from build123d import *

# Parameters (mm, degrees)
CROQUIS1_R              = 12
CROQUIS1_R_2            = 1.7
SALIENTE_EXTRUIR1_DEPTH = 10
CROQUIS2_R              = 4
SALIENTE_EXTRUIR2_DEPTH = 20
CORTAR_EXTRUIR1_REACH   = 12
CROQUIS3_R              = 5.5


with BuildPart() as part:
    # Croquis1 → Saliente-Extruir1 (new body)
    with BuildSketch(Plane.XY):
        Circle(CROQUIS1_R)
        with Locations((-5.655, 5.655)):
            Circle(CROQUIS1_R_2, mode=Mode.SUBTRACT)
        with Locations((5.655, 5.655)):
            Circle(CROQUIS1_R_2, mode=Mode.SUBTRACT)
        with Locations((5.655, -5.655)):
            Circle(CROQUIS1_R_2, mode=Mode.SUBTRACT)
        with Locations((-5.655, -5.655)):
            Circle(CROQUIS1_R_2, mode=Mode.SUBTRACT)
    extrude(amount=SALIENTE_EXTRUIR1_DEPTH)

    # Croquis2 → Saliente-Extruir2 (add, symmetric)
    with BuildSketch(Plane(origin=(0, 0, 0), x_dir=(0, 0, -1), z_dir=(1, 0, 0))):
        with Locations((-4, 0)):
            Circle(CROQUIS2_R)
    extrude(amount=SALIENTE_EXTRUIR2_DEPTH, both=True)

    # Croquis3 → Cortar-Extruir1 (cut, up to next)
    with BuildSketch(Plane.XY.offset(10), mode=Mode.PRIVATE) as cortar_extruir1_sk1:
        Circle(CROQUIS3_R)
    cortar_extruir1_tool1 = extrude(cortar_extruir1_sk1.sketch, amount=-CORTAR_EXTRUIR1_REACH, mode=Mode.PRIVATE) & part.part
    add(cortar_extruir1_tool1.solids().sort_by_distance((0, 0, 10))[0], mode=Mode.SUBTRACT)


solid = part.part
Build history of the part. All positions in model axes, mm. A direction names the side the tool comes from. Give positions to 0.01 mm unless a question says otherwise; leave off trailing zeros. Loops run counter-clockwise (first coordinate to the right, second up) from the corner with the lowest first, then second, coordinate; pieces in that order, holes last. Notation, with made-up numbers: (49, 80.25) - (97, 80.25) arc R22 ccw to (97, 118.25) - close; hole circle Ø1 at (50, 42). An arc over 180 degrees is marked (long way). Write item = value, one per line. Start each with the question number.
1) Probe probe 1 along X at (y, z) = (4.75, 6.75); probe 2 along Y at (x, z) = (-5, 3); probe 3 along X at (y, z) = (-4.25, 5.25). List the from-to ranges inside material, lowest first. Write a range as from..to.
2) Band-saw the part on B-B on z = 4. Give the cut face in (x, y) (3 decimals).
3) Band-saw the part on D-D on z = 7.5. Give the cut face in (x, y) (1 decimal).
4) Tool access for faces 1 (the cylindrical face through (-1.19, -5.37, 5.07)), 2 (the cylindrical face through (-15.596, 3.966, 4.521)): list every direction of +Z, -Z, +X, -X, +Y, -Y with a clear straight run to the whole face (end or side of a thin tool).
5) Pull direction X, two halves, no side cores. Call faces 3 (the flat face through (20, 0, 4)), 4 (the cylindrical face through (16, 0, 8)), 5 (the cylindrical face through (-5.88, 7.34, 4.93)): +X half, -X half, draft (parallel to the pull), parting line (faces both ways), or undercut.
6) Band-saw the part on C-C on y = -1. Give the cut face in (x, z), plus the area to 3 significant figures.
7) Drop flat-ended pins along their axis: pin 1 Ø5.5 at (x, y) = (5.655, 5.655) entering from +Z; pin 2 Ø6 at (x, z) = (-4, 3.5) entering from +Y; pin 3 Ø1 at (x, z) = (-13, 8) entering from -Y; pin 4 Ø3 at (x, z) = (2.5, 7) entering from -Y. Give the stop position or say it passes through.
8) Band-saw the part on A-A on x = 0. Give the cut face in (y, z).
Final values:
q1.probe_1 = -11.02..-7.09, -4.22..-2.77, 2.77..4.22, 7.09..11.02
q1.probe_2 = -10.91..-7.22, -4.09..-2.29, 2.29..4.09, 7.22..10.91
q1.probe_3 = -11.22..-6.61, -4.7..-3.49, 3.49..4.7, 6.61..11.22
q2.outline = (-20, -4) - (-11.314, -4) arc R12 ccw to (11.314, -4) - (20, -4) - (20, 4) - (11.314, 4) arc R12 ccw to (-11.314, 4) - (-20, 4) - close; hole (-6.044, -4) arc R1.7 ccw (long way) to (-5.266, -4) - close; hole (-6.044, 4) - (-5.266, 4) arc R1.7 ccw (long way) to start; hole circle Ø11 at (0, 0); hole (5.266, -4) arc R1.7 ccw (long way) to (6.044, -4) - close; hole (5.266, 4) - (6.044, 4) arc R1.7 ccw (long way) to start
q3.outline = (-20, -1.9) - (-11.8, -1.9) arc R12 ccw to (11.8, -1.9) - (20, -1.9) - (20, 1.9) - (11.8, 1.9) arc R12 ccw to (-11.8, 1.9) - (-20, 1.9) - close; hole circle Ø3.4 at (-5.7, -5.7); hole circle Ø3.4 at (-5.7, 5.7); hole circle Ø11 at (0, 0); hole circle Ø3.4 at (5.7, -5.7); hole circle Ø3.4 at (5.7, 5.7)
q4.face_1 = +Z, -Z
q4.face_2 = -X
q5.face_3 = +X half
q5.face_4 = draft
q5.face_5 = undercut
q6.outline = (-20, 0.13) - (-11.96, 0.13) - (-11.96, 0) - (-5.41, 0) - (-5.41, 10) - (-11.96, 10) - (-11.96, 7.87) - (-20, 7.87) - close; (5.41, 0) - (11.96, 0) - (11.96, 0.13) - (20, 0.13) - (20, 7.87) - (11.96, 7.87) - (11.96, 10) - (5.41, 10) - close
q6.area = 256 mm²
q7.pin_1 = 10
q7.pin_2 = 11.96
q7.pin_3 = -1.94
q7.pin_4 = -11.96
q8.outline = (-12, 0) - (-5.5, 0) - (-5.5, 10) - (-12, 10) - close; (5.5, 0) - (12, 0) - (12, 10) - (5.5, 10) - close
